Can you work these out from the model? Positions are in its coordinate system, mm. A direction names the side the tool comes from. Coordinates: 2 decimals unless noted, no trailing zeros. Order: outer loops, then holes, each group sorted by start corner. A loop starts at its lowest first (then second) coordinate and runs counter-clockwise, first axis right, second up. Notation, with made-up numbers: (44.25, 23.5) -> (85.25, 23.5) arc R20 cw to (85.25, 60.5) -> close; hole circle Ø1 at (71.5, 75.5). An arc over 180 degrees is marked (long way). Use a Markdown table: item, result. Add a question column.
1. Suppose I cut it at A-A, the plane y = 0. List the corners of the cut face in (x, z) for me (3 decimals).
2. For pin 1 Ø1.5 at (x, y) = (29, 5.5) entering from +Z; pin 2 Ø6 at (x, y) = (-4, 8) entering from +Z; pin 3 Ø2 at (x, y) = (3.5, 9) entering from -Z, each with a flat end and sliding along its axis, tell me the tip position at first contact or that it passes through.
3. If I drill on line 1 along Y through (x, z) = (-3, 0) (3 decimals); line 2 along Y through (x, z) = (28.25, 0) (3 decimals); line 3 along Z through (x, y) = (4.5, 0.5), over which ranges is the centre line in solid material (lowest first)? Write a range as from..to.
4. We'd pull the mould along Y, two halves only. Please class faces 4 (the cylindrical face through (29.1, -7.52, -8.2)), 5 (the conical face through (22.14, 8.8, -11.48)), 6 (the flat face through (-10, -17.3, -0.1)): pulls with the +Y half, pulls with the -Y half, needs draft (parallel to the pull), parting line crosses it, or undercut.
5. Suppose I cut it at C-C, the plane x = -6.5. List the corners of the cut face in (y, z) for me (3 decimals), then the cut area to 3 significant figures.
6. Suppose I cut it at D-D, the plane x = 30.5. List the corners of the cut face in (y, z) for me (3 decimals), then the cut area to 3 significant figures.
7. For faces 1 (the cylindrical face through (29.29, -4.243, 13.473)), 2 (the cylindrical face through (1.22, -7.5, 18.08)), 3 (the flat face through (0, -16.55, -2.61)), which set-ups out of +Z, -Z, +X, -X, +Y, -Y let a thin tool reach every point of the face, with its end or its side?
```python
from build123d import *

# Parameters (mm, degrees)
BOSS_EXTRUDE1_START = 10
SKETCH2_R           = 19.575
SKETCH2_R_2         = 17.1
BOSS_EXTRUDE1_DEPTH = 10


with BuildPart() as part:
    # Sketch1 → Revolve1 (revolve)
    with BuildSketch(Plane(origin=(0, 0, 0), x_dir=(1, 0, 0), z_dir=(0, 1, 0)), mode=Mode.PRIVATE) as revolve1_sk:
        Polygon((0, 16.575), (12, 16.575), (22, 11.125), (36, 11.125), (36, 14.125), (22.764422316, 14.125), (12.764422316, 19.575), (0, 19.575), align=None)
    revolve(revolve1_sk.sketch.rotate(Axis((0, 0, 0), (1, 0, 0)), 180), axis=Axis((0, 0, 0), (1, 0, 0)))

    # Sketch2 → Boss-Extrude1 (add)
    with BuildSketch(Plane.ZY.offset(BOSS_EXTRUDE1_START)):
        Circle(SKETCH2_R)
        Circle(SKETCH2_R_2, mode=Mode.SUBTRACT)
    extrude(amount=-BOSS_EXTRUDE1_DEPTH)


solid = part.part
```
Worked out:
| question | item | result |
|---|---|---|
| 1 | outline | (-10, -19.575) -> (12.764, -19.575) -> (22.764, -14.125) -> (36, -14.125) -> (36, -11.125) -> (22, -11.125) -> (12, -16.575) -> (0, -16.575) -> (0, -17.1) -> (-10, -17.1) -> close; (-10, 17.1) -> (0, 17.1) -> (0, 16.575) -> (12, 16.575) -> (22, 11.125) -> (36, 11.125) -> (36, 14.125) -> (22.764, 14.125) -> (12.764, 19.575) -> (-10, 19.575) -> close |
| 2 | pin 1 | stops at z = 13.3 |
| 2 | pin 2 | stops at z = 18.93 |
| 2 | pin 3 | stops at z = -17.87 |
| 3 | line 1 | y = -19.575..-17.1, 17.1..19.575 |
| 3 | line 2 | y = -14.125..-11.125, 11.125..14.125 |
| 3 | line 3 | z = -19.57..-16.57, 16.57..19.57 |
| 4 | face 4 | undercut |
| 4 | face 5 | parting line crosses it |
| 4 | face 6 | needs draft |
| 5 | outline | circle Ø39.15 at (0, 0); hole circle Ø34.2 at (0, 0) |
| 5 | area | 285 mm² |
| 6 | outline | circle Ø28.25 at (0, 0); hole circle Ø22.25 at (0, 0) |
| 6 | area | 238 mm² |
| 7 | face 1 | +X |
| 7 | face 2 | +X, -X |
| 7 | face 3 | -X |
